from build123d import *

# Parameters (mm, degrees)
ESQUISSE1_W                = 60
ESQUISSE1_H                = 50
BOSS_EXTRU_1_DEPTH         = 15
BOSS_EXTRU_2_DEPTH         = 50
ESQUISSE3_R                = 4.5
ESQUISSE3_R_2              = 3.25
BOSS_EXTRU_3_DEPTH         = 1
ESQUISSE4_R                = 2.75
ENL_V_MAT_EXTRU_1_DEPTH    = 50
ESQUISSE5_R                = 2.5
ENL_V_MAT_EXTRU_2_DEPTH    = 15
R_P_TITION_LIN_AIRE1_COUNT = 2
R_P_TITION_LIN_AIRE1_PITCH = 30
R_P_TITION_LIN_AIRE2_COUNT = 2
R_P_TITION_LIN_AIRE2_PITCH = 40


with BuildPart() as part:
    # Esquisse1 → Boss.-Extru.1 (new body)
    with BuildSketch(Plane.XY):
        Rectangle(ESQUISSE1_W, ESQUISSE1_H)
    extrude(amount=BOSS_EXTRU_1_DEPTH)

    # Esquisse2 → Boss.-Extru.2 (add)
    with BuildSketch(Plane(origin=(0, 25, 0), x_dir=(1, 0, 0), z_dir=(0, 1, 0))):
        with BuildLine():
            Line((-7.5, -15), (7.5, -15))
            ThreePointArc((7.5, -15), (0, -22.5), (-7.5, -15))
        make_face()
    extrude(amount=-BOSS_EXTRU_2_DEPTH)

    # Esquisse3 → Boss.-Extru.3 (add)
    with BuildSketch(Plane(origin=(0, 25, 0), x_dir=(1, 0, 0), z_dir=(0, 1, 0))):
        with Locations((0, -15)):
            Circle(ESQUISSE3_R)
        with Locations((0, -15)):
            Circle(ESQUISSE3_R_2, mode=Mode.SUBTRACT)
    extrude(amount=BOSS_EXTRU_3_DEPTH)

    # Esquisse4 → Enlèv. mat.-Extru.1 (cut)
    with BuildSketch(Plane(origin=(0, 25, 0), x_dir=(1, 0, 0), z_dir=(0, 1, 0))):
        with Locations((0, -15)):
            Circle(ESQUISSE4_R)
    extrude(amount=-ENL_V_MAT_EXTRU_1_DEPTH, mode=Mode.SUBTRACT)

    # Esquisse5 → Enlèv. mat.-Extru.2 (cut)
    with BuildSketch(Plane.XY.offset(15)):
        with Locations((-20, -15)):
            Circle(ESQUISSE5_R)
        with Locations((-20, 15)):
            Circle(ESQUISSE5_R)
        with Locations((20, -15)):
            Circle(ESQUISSE5_R)
        with Locations((20, 15)):
            Circle(ESQUISSE5_R)
    extrude(amount=-ENL_V_MAT_EXTRU_2_DEPTH, mode=Mode.SUBTRACT)

    # Esquisse13 → Enlèvement de matière-Révolution1 (revolve, cut)
    with BuildSketch(Plane.XZ.offset(15)):
        Polygon((-24.5, 15), (-22.5, 13), (-22.5, 15), align=None)
    enl_vement_de_mati_re_r_volution1 = revolve(axis=Axis((-20, -15, 15), (0, 0, -1)), mode=Mode.SUBTRACT)

    # Répétition linéaire1: Enlèvement de matière-Révolution1 ×2
    with Locations(*[(0, i * R_P_TITION_LIN_AIRE1_PITCH, 0) for i in range(1, R_P_TITION_LIN_AIRE1_COUNT)]):
        add(enl_vement_de_mati_re_r_volution1, mode=Mode.SUBTRACT)

    # Répétition linéaire2: Enlèvement de matière-Révolution1 ×2
    with Locations(*[(i * R_P_TITION_LIN_AIRE2_PITCH, 0, 0) for i in range(1, R_P_TITION_LIN_AIRE2_COUNT)]):
        add(enl_vement_de_mati_re_r_volution1, mode=Mode.SUBTRACT)

    # Répétition linéaire2 copy 1 sketch → Répétition linéaire2 copy 1 (revolve, cut)
    with BuildSketch(Plane(origin=(40, 15, 0), x_dir=(1, 0, 0), z_dir=(0, -1, 0))):
        Polygon((-24.5, 15), (-22.5, 13), (-22.5, 15), align=None)
    revolve(axis=Axis((20, 15, 15), (0, 0, -1)), mode=Mode.SUBTRACT)


solid = part.part
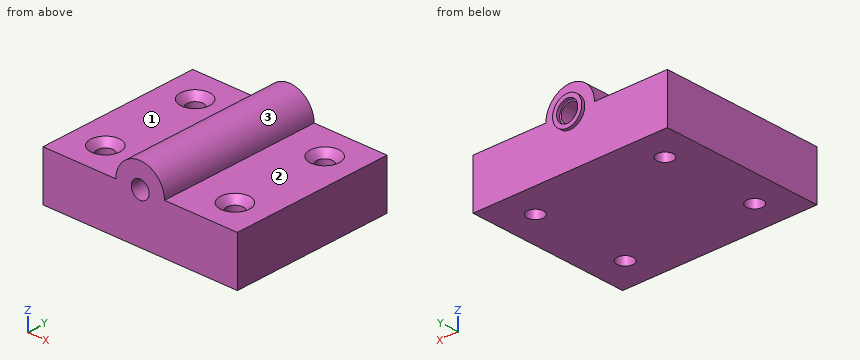
Design review of the part built by this model. Coordinates are the model's own, in mm. Face numbers are marked on the shaded views. A direction names the side the tool comes from. Round coordinates to 2 decimals unless told otherwise and drop trailing zeros. Write each loop counter-clockwise with the first axis right and the second up, starting at its lowest first coordinate (ties: lowest second). Pieces come first, ordered by that corner, then holes.
Item 1: Consider section A-A on y = 15. Give the boundary of the cut face in (x, z), and give its area (3 significant figures).
Item 2: Consider section B-B on x = -20. Give the boundary of the cut face in (y, z).
Item 3: Consider section D-D on x = 0. Give the boundary of the cut face in (y, z).
Item 4: Wall thickness on L1, parallel to X at y = 15, z = 4.25; L2, parallel to Y at x = 20, z = 8.75; L3, parallel to Z at x = 0, y = 25.45: over which ranges is each line inside the solid? List them lowest first.
Item 5: For pin 1 Ø11 at (x, y) = (-13.5, -11) entering from +Z; pin 2 Ø3 at (y, z) = (17, 17.5) entering from +X; pin 3 Ø11 at (x, z) = (-14, 7) entering from +Y; pin 4 Ø12 at (x, y) = (-1, 15) entering from -Z, all flat-tipped, find the tip position at first contact; note any pin that passes through.
Item 6: For the marked faces 1, 2 and 3, list the 3-axis set-ups (+Z, -Z, +X, -X, +Y, -Y) from which the entire face can be reached by the end or side of a thin tool; tool diameter is ignored.
Item 7: Consider section C-C on z = 14.25. Give the boundary of the cut face in (x, y).
Check values:
1. outline: (-30, 0) - (-22.5, 0) - (-22.5, 13) - (-24.5, 15) - (-30, 15) - close; (-17.5, 0) - (17.5, 0) - (17.5, 13) - (15.5, 15) - (7.5, 15) arc R7.5 ccw to (-7.5, 15) - (-15.5, 15) - (-17.5, 13) - close; (22.5, 0) - (30, 0) - (30, 15) - (24.5, 15) - (22.5, 13) - close; hole circle Ø5.5 at (0, 15)
1. area: 807 mm2
2. outline: (-25, 0) - (-17.5, 0) - (-17.5, 13) - (-19.5, 15) - (-25, 15) - close; (-12.5, 0) - (12.5, 0) - (12.5, 13) - (10.5, 15) - (-10.5, 15) - (-12.5, 13) - close; (17.5, 0) - (25, 0) - (25, 15) - (19.5, 15) - (17.5, 13) - close
3. outline: (-25, 0) - (25, 0) - (25, 10.5) - (26, 10.5) - (26, 11.75) - (25, 11.75) - (25, 12.25) - (-25, 12.25) - close; (-25, 17.75) - (25, 17.75) - (25, 18.25) - (26, 18.25) - (26, 19.5) - (25, 19.5) - (25, 22.5) - (-25, 22.5) - close
4. L1: x = -30 to -22.5, -17.5 to 17.5, 22.5 to 30
4. L2: y = -25 to -17.5, -12.5 to 12.5, 17.5 to 25
4. L3: z = 10.5 to 11.75, 18.25 to 19.5
5. pin 1: stops at z = 15
5. pin 2: stops at x = 7.43
5. pin 3: stops at y = 25
5. pin 4: stops at z = 0
6. face 1: +Z, -X, +Y, -Y
6. face 2: +Z, +X, +Y, -Y
6. face 3: +Z, +Y, -Y
7. outline: (-30, -25) - (-2.65, -25) - (-2.65, 25) - (-3.16, 25) - (-3.16, 26) - (-4.44, 26) - (-4.44, 25) - (-30, 25) - close; (2.65, -25) - (30, -25) - (30, 25) - (4.44, 25) - (4.44, 26) - (3.16, 26) - (3.16, 25) - (2.65, 25) - close; hole circle Ø7.5 at (-20, -15); hole circle Ø7.5 at (-20, 15); hole circle Ø7.5 at (20, -15); hole circle Ø7.5 at (20, 15)
